from build123d import *

# Parameters (mm, degrees)
F0_R     = 63.008602
F1_DEPTH = 25.4
F2_R     = 13.792903
F3_DEPTH = 63.5
F4_R     = 22.697716
F5_DEPTH = 12.7
F6_R     = 17.487641
F7_DEPTH = 127


with BuildPart() as f1:
    # F0 (on Front) → F1 (new body)
    with BuildSketch(Plane.XZ):
        Circle(F0_R)
    extrude(amount=F1_DEPTH)

    # F2 (on Front) → F3 (join)
    with BuildSketch(Plane.XZ):
        with Locations((0, 35.29866)):
            Circle(F2_R)
    extrude(amount=F3_DEPTH)

    # F4 (on face) → F5 (join)
    with BuildSketch(Plane.XZ.offset(63.5)):
        with Locations((0, 35.29866)):
            Circle(F4_R)
    extrude(amount=-F5_DEPTH)

    # F6 (on face) → F7 (join)
    with BuildSketch(Plane(origin=(0, 0, 0), x_dir=(-1, 0, 0), z_dir=(0, 1, 0))):
        Circle(F6_R)
    extrude(amount=F7_DEPTH)


solid = f1.part
Check sheet for the modelled part. Datum: model origin and axes. Units: mm. A direction names the side the tool comes from. Give positions to 0.01 mm unless a question says otherwise; leave off trailing zeros. Write each loop counter-clockwise with the first axis right and the second up, starting at its lowest first coordinate (ties: lowest second). Pieces come first, ordered by that corner, then holes. Notation, with made-up numbers: (-14, 3) -> (32, 3) arc R31 cw to (32, 27) -> close; hole circle Ø10 at (55, 38.25). An arc over 180 degrees is marked (long way). One line per item, written item: value. Start each with the question number.
Item 1: Section check A-A on z = 0. Record the cut outline in (x, y).
Item 2: Section check B-B on x = 0. Record the cut outline in (y, z), then the cut area to 3 significant figures.
Item 3: Tool access check on faces 1 (the flat face through (0, 127, 0)), 2 (the cylindrical face through (2.28, 62.61, 17.34)), 3 (the cylindrical face through (12.2, -57.24, 54.44)). Record the directions out of +Z, -Z, +X, -X, +Y, -Y that give a thin tool (end or side, any length) a straight path to the whole face; none if there is none.
Item 4: Draft check along Y on faces 4 (the flat face through (13, 0, -13)), 5 (the cylindrical face through (-13.7, -12.5, -61.5)), 6 (the cylindrical face through (-2.99, -37.922, 21.834)), 7 (the flat face through (0, -50.8, 20)). Enter one of: +Y half, -Y half, draft (parallel to the pull), parting line (faces both ways), or undercut.
Item 5: Section check C-C on y = -19.5. Record the cut outline in (x, z), then the cut area to 3 significant figures.
Item 6: Gauge pin test, flat ends, axial feed: pin 1 (10 mm diameter, centred on y = 91, z = 8, fed in from +X); pin 2 (10 mm diameter, centred on x = -38, z = 45.5, fed in from -Y); pin 3 (8 mm diameter, centred on x = -5, y = 29.5, fed in from -Z). Record the tip position at first contact, or that the pin passes through.
Item 7: Material ranges on probe 1 along Y at (x, z) = (5, 50); probe 2 along Y at (x, z) = (-4, 30); probe 3 along X at (y, z) = (16.5, 1), recorded low to high. Write a range as from..to.
Item 8: Section check D-D on z = 29.5. Record the cut outline in (x, y), then the cut area to 3 significant figures.
Results list:
1. outline: (-63.01, -25.4) -> (63.01, -25.4) -> (63.01, 0) -> (17.49, 0) -> (17.49, 127) -> (-17.49, 127) -> (-17.49, 0) -> (-63.01, 0) -> close
2. outline: (-63.5, 12.6) -> (-50.8, 12.6) -> (-50.8, 21.51) -> (-25.4, 21.51) -> (-25.4, -63.01) -> (0, -63.01) -> (0, -17.49) -> (127, -17.49) -> (127, 17.49) -> (0, 17.49) -> (0, 63.01) -> (-25.4, 63.01) -> (-25.4, 49.09) -> (-50.8, 49.09) -> (-50.8, 58) -> (-63.5, 58) -> close
2. area: 8,920 mm²
3. face 1: +Z, -Z, +X, -X, +Y
3. face 2: +Y
3. face 3: -Y
4. face 4: +Y half
4. face 5: draft
4. face 6: undercut
4. face 7: undercut
5. outline: circle Ø126.02 at (0, 0)
5. area: 12,500 mm²
6. pin 1: x = 17.23
6. pin 2: y = -25.4
6. pin 3: z = -17.46
7. probe 1: -63.5..-50.8, -25.4..0
7. probe 2: -63.5..0
7. probe 3: -17.46..17.46
8. outline: (-55.68, -25.4) -> (-12.51, -25.4) -> (-12.51, -50.8) -> (-21.94, -50.8) -> (-21.94, -63.5) -> (21.94, -63.5) -> (21.94, -50.8) -> (12.51, -50.8) -> (12.51, -25.4) -> (55.68, -25.4) -> (55.68, 0) -> (-55.68, 0) -> close
8. area: 4,020 mm²
